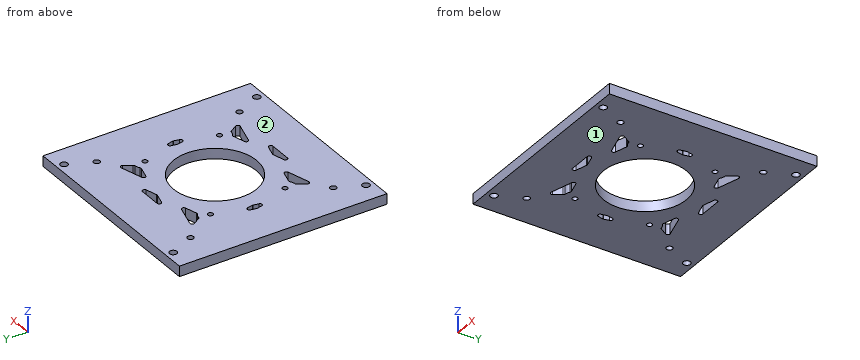
from build123d import *

# Parameters (mm, degrees)
SKETCH_1_W          = 100
SKETCH_1_H          = 100
EXTRUDE_1_DEPTH     = 5
SKETCH_2_R          = 1.75
CUT_EXTRUDE_1_DEPTH = 5
SKETCH_3_R          = 1.25
SKETCH_3_R_2        = 1.5
SKETCH_3_R_3        = 20
CUT_EXTRUDE_2_DEPTH = 5
CUT_EXTRUDE_3_DEPTH = 5
FILLET_27_R         = 1


with BuildPart() as part:
    # 草图1 → 凸台-拉伸1 (new body)
    with BuildSketch(Plane.XY):
        with Locations((50, 50)):
            Rectangle(SKETCH_1_W, SKETCH_1_H)
    extrude(amount=EXTRUDE_1_DEPTH)

    # 草图2 → 切除-拉伸1 (cut)
    with BuildSketch(Plane.XY.offset(5)):
        with Locations((10, 96.45)):
            Circle(SKETCH_2_R)
        with Locations((90, 96.45)):
            Circle(SKETCH_2_R)
        with Locations((10, 3.55)):
            Circle(SKETCH_2_R)
        with Locations((90, 3.55)):
            Circle(SKETCH_2_R)
    extrude(amount=-CUT_EXTRUDE_1_DEPTH, mode=Mode.SUBTRACT)

    # 草图3 → 切除-拉伸2 (cut)
    with BuildSketch(Plane.XY.offset(5)):
        with Locations((26, 68)):
            Circle(SKETCH_3_R)
        with Locations((74, 68)):
            Circle(SKETCH_3_R)
        with Locations((26, 32)):
            Circle(SKETCH_3_R)
        with Locations((74, 32)):
            Circle(SKETCH_3_R)
        with Locations((15.6, 84.4)):
            Circle(SKETCH_3_R_2)
        with Locations((84.4, 84.4)):
            Circle(SKETCH_3_R_2)
        with Locations((84.4, 15.6)):
            Circle(SKETCH_3_R_2)
        with Locations((15.6, 15.6)):
            Circle(SKETCH_3_R_2)
        with Locations((50, 50)):
            Circle(SKETCH_3_R_3)
    extrude(amount=-CUT_EXTRUDE_2_DEPTH, mode=Mode.SUBTRACT)

    # 草图4 → 切除-拉伸3 (cut)
    with BuildSketch(Plane.XY.offset(5)):
        Polygon((62.620906011, 81.4), (37.379093989, 81.4), (50, 77.85577297), align=None)
        with BuildLine():
            Line((38.90383284, 74.739726027), (22.326209721, 79.395085944))
            Line((22.326209721, 79.395085944), (26.226184699, 73.245125402))
            ThreePointArc((26.226184699, 73.245125402), (27.87858351, 72.902389621), (29.336878066, 72.05311544))
            Line((29.336878066, 72.05311544), (38.90383284, 74.739726027))
        make_face()
        with BuildLine():
            Line((77.673790279, 79.395085944), (61.09616716, 74.739726027))
            Line((61.09616716, 74.739726027), (70.663121934, 72.05311544))
            ThreePointArc((70.663121934, 72.05311544), (72.12141649, 72.902389621), (73.773815301, 73.245125402))
            Line((73.773815301, 73.245125402), (77.673790279, 79.395085944))
        make_face()
        Polygon((50, 22.14422703), (37.379093989, 18.6), (62.620906011, 18.6), align=None)
        with BuildLine():
            ThreePointArc((29.336878066, 27.94688456), (27.87858351, 27.097610379), (26.226184699, 26.754874598))
            Line((26.226184699, 26.754874598), (22.326209721, 20.604914056))
            Line((22.326209721, 20.604914056), (38.90383284, 25.260273973))
            Line((38.90383284, 25.260273973), (29.336878066, 27.94688456))
        make_face()
        with BuildLine():
            Line((70.663121934, 27.94688456), (61.09616716, 25.260273973))
            Line((61.09616716, 25.260273973), (77.673790279, 20.604914056))
            Line((77.673790279, 20.604914056), (73.773815301, 26.754874598))
            ThreePointArc((73.773815301, 26.754874598), (72.12141649, 27.097610379), (70.663121934, 27.94688456))
        make_face()
        Polygon((22.427480916, 50), (20.898222534, 57.70510954), (19.368964152, 50), (20.898222534, 42.29489046), align=None)
        Polygon((79.101777466, 42.29489046), (80.631035848, 50), (79.101777466, 57.70510954), (77.572519084, 50), align=None)
    extrude(amount=-CUT_EXTRUDE_3_DEPTH, mode=Mode.SUBTRACT)

    # 圆角27
    fillet_27_edges = [part.edges().sort_by_distance(p)[0] for p in [
        (29.336878066, 72.05311544, 2.5),
        (26.226184699, 73.245125402, 2.5),
        (22.326209721, 79.395085944, 2.5),
        (38.90383284, 74.739726027, 2.5),
        (73.773815301, 73.245125402, 2.5),
        (70.663121934, 72.05311544, 2.5),
        (61.09616716, 74.739726027, 2.5),
        (77.673790279, 79.395085944, 2.5),
        (26.226184699, 26.754874598, 2.5),
        (29.336878066, 27.94688456, 2.5),
        (38.90383284, 25.260273973, 2.5),
        (22.326209721, 20.604914056, 2.5),
        (50, 22.14422703, 2.5),
        (62.620906011, 18.6, 2.5),
        (37.379093989, 18.6, 2.5),
        (79.101777466, 57.70510954, 2.5),
        (80.631035848, 50, 2.5),
        (79.101777466, 42.29489046, 2.5),
        (77.572519084, 50, 2.5),
        (20.898222534, 42.29489046, 2.5),
        (19.368964152, 50, 2.5),
        (20.898222534, 57.70510954, 2.5),
        (22.427480916, 50, 2.5),
        (70.663121934, 27.94688456, 2.5),
        (73.773815301, 26.754874598, 2.5),
        (77.673790279, 20.604914056, 2.5),
        (61.09616716, 25.260273973, 2.5),
        (50, 77.85577297, 2.5),
        (37.379093989, 81.4, 2.5),
        (62.620906011, 81.4, 2.5),
    ]]
    fillet(fillet_27_edges, radius=FILLET_27_R)


solid = part.part
Can you work these out from the model? Positions are in its coordinate system, mm. Face numbers are marked on the shaded views. Give positions to 0.01 mm unless a question says otherwise; leave off trailing zeros. Order: outer loops, then holes, each group sorted by start corner. A loop starts at its lowest first (then second) coordinate and runs counter-clockwise, first axis right, second up. Notation, with made-up numbers: M -33,40 L 21,40 A13 ccw 21,55 Z; hole C 35.5,85 d9. An arc over 180 degrees is marked long. Use one line per item in the form item = value.
Item 1: Thinking about a two-plate mould opening in Z: for the marked faces 1 and 2, which applies, pulls with the +Z half, pulls with the -Z half, needs draft (parallel to the pull), parting line crosses it, or undercut?
Values follow:
face_1 = pulls with the -Z half
face_2 = pulls with the +Z half
Item 2: If we section it at C-C, the plane y = 44: Write out the boundary of the cut face in (x, z), and give its area (3 significant figures).
Values follow:
outline = M 0,0 L 30.92,0 L 30.92,5 L 0,5 Z; M 69.08,0 L 100,0 L 100,5 L 69.08,5 Z
area = 309 mm^2
Item 3: If we section it at A-A, the plane x = 90: Write out the boundary of the cut face in (y, z).
Values follow:
outline = M 0,0 L 1.8,0 L 1.8,5 L 0,5 Z; M 5.3,0 L 94.7,0 L 94.7,5 L 5.3,5 Z; M 98.2,0 L 100,0 L 100,5 L 98.2,5 Z
Item 4: Will these pins go through, and if not, where does the flat tip stop? pin 1 Ø3 at (x, y) = (26, 68) entering from +Z; pin 2 Ø1.8 at (x, y) = (84.4, 84.4) entering from -Z.
Values follow:
pin_1 = 5
pin_2 = through
Item 5: If we section it at B-B, the plane y = 84.4: Write out the boundary of the cut face in (x, z).
Values follow:
outline = M 0,0 L 14.1,0 L 14.1,5 L 0,5 Z; M 17.1,0 L 82.9,0 L 82.9,5 L 17.1,5 Z; M 85.9,0 L 100,0 L 100,5 L 85.9,5 Z
Item 6: If we section it at D-D, the plane x = 41: Write out the boundary of the cut face in (y, z).
Values follow:
outline = M 0,0 L 32.14,0 L 32.14,5 L 0,5 Z; M 67.86,0 L 100,0 L 100,5 L 67.86,5 Z
Item 7: If I drill on line 1 along X through (y, z) = (84.4, 1.1); line 2 along Y through (x, z) = (51, 1.7), over which ranges is the centre line in solid material (lowest first)? Write a range as [from, to].
Values follow:
line_1 = [0, 14.1], [17.1, 82.9], [85.9, 100]
line_2 = [0, 18.6], [21.86, 30.03], [69.97, 78.14], [81.4, 100]
